from build123d import *

# Parameters (mm, degrees)
SKETCH1_R           = 161.29
BOSS_EXTRUDE1_DEPTH = 161.29
SKETCH3_W           = 4310.634
SKETCH3_H           = 18064.48
SKETCH3_R           = 161.29
BOSS_EXTRUDE3_DEPTH = 161.29
SCALE2_SCALE        = 0.039370079


with BuildPart() as part:
    # Sketch1 → Boss-Extrude1 (new body)
    with BuildSketch(Plane.XY):
        Polygon((-2155.317, 3225.8), (3592.046917484, 8973.163917484), (5747.419448428, 6817.902448428), (2155.317, 3225.8), (2155.317, -3225.8), (-2155.317, -3225.8), align=None)
        with Locations((4804.833357851, 7304.254711836)):
            Circle(SKETCH1_R, mode=Mode.SUBTRACT)
        with Locations((3892.43933595, 6391.860689935)):
            Circle(SKETCH1_R, mode=Mode.SUBTRACT)
        with Locations((2980.04531405, 5479.466668034)):
            Circle(SKETCH1_R, mode=Mode.SUBTRACT)
        with Locations(Location((2253.753739605, 6205.720818177, 0), (0, 0, 180))):
            Circle(SKETCH1_R, mode=Mode.SUBTRACT)
        with Locations(Location((3166.100745307, 7118.161853854, 0), (0, 0, 180))):
            Circle(SKETCH1_R, mode=Mode.SUBTRACT)
        with Locations(Location((4078.447751009, 8030.602889531, 0), (0, 0, 180))):
            Circle(SKETCH1_R, mode=Mode.SUBTRACT)
    extrude(amount=-BOSS_EXTRUDE1_DEPTH)

    # Sketch3 → Boss-Extrude3 (add)
    with BuildSketch(Plane(origin=(0, -3225.8, 0), x_dir=(-1, 0, 0), z_dir=(0, -1, 0))):
        with Locations((0, 9032.24)):
            Rectangle(SKETCH3_W, SKETCH3_H)
        with BuildLine():
            ThreePointArc((-1076.325000002, 3548.374999923), (-961.455647452, 3501.587385122), (-913.765000004, 3387.09))
            ThreePointArc((-913.765000004, 3387.09), (-961.455647452, 3272.592614878), (-1076.325000002, 3225.805000077))
            ThreePointArc((-1076.325000002, 3225.805000077), (-1238.885, 3387.09), (-1076.325000002, 3548.374999923))
        make_face(mode=Mode.SUBTRACT)
        with Locations(Location((1075.054999996, 3387.089999999, 0), (0, 0, 180))):
            Circle(SKETCH3_R, mode=Mode.SUBTRACT)
        with BuildLine():
            ThreePointArc((-1076.325000001, 10322.565000077), (-1238.885, 10483.85), (-1076.325, 10645.134999923))
            ThreePointArc((-1076.325, 10645.134999923), (-961.455647452, 10598.347385122), (-913.765000004, 10483.85))
            ThreePointArc((-913.765000004, 10483.85), (-961.455647452, 10369.352614878), (-1076.325000001, 10322.565000077))
        make_face(mode=Mode.SUBTRACT)
        with BuildLine():
            ThreePointArc((-1076.325000002, 17419.325000077), (-1238.885, 17580.61), (-1076.325000002, 17741.894999923))
            ThreePointArc((-1076.325000002, 17741.894999923), (-961.455647452, 17695.107385122), (-913.765000004, 17580.61))
            ThreePointArc((-913.765000004, 17580.61), (-961.455647452, 17466.112614878), (-1076.325000002, 17419.325000077))
        make_face(mode=Mode.SUBTRACT)
        with Locations(Location((1077.594999996, 10483.849999999, 0), (0, 0, 180))):
            Circle(SKETCH3_R, mode=Mode.SUBTRACT)
        with Locations(Location((1077.595, 17580.609999999, 0), (0, 0, 180))):
            Circle(SKETCH3_R, mode=Mode.SUBTRACT)
    extrude(amount=BOSS_EXTRUDE3_DEPTH)


with BuildPart() as part_1:
    # Scale2: scaled about (342.584657251, -1172.717670217, -5623.777851714)
    add(part.part.scale(SCALE2_SCALE).moved(Location((329.09707232, -1126.547683201, -5402.369274875))))


solid = part_1.part
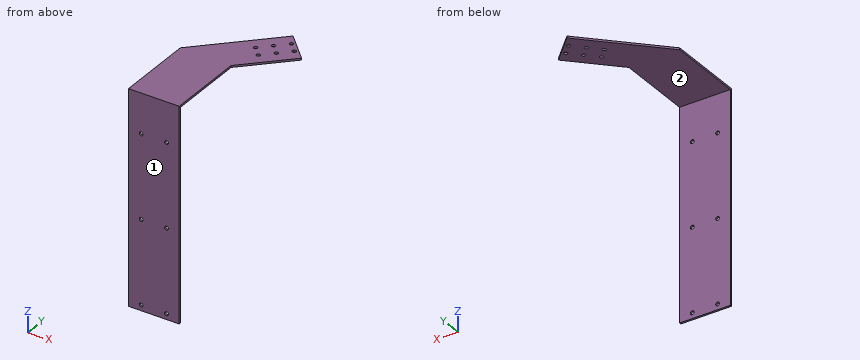
Read the model definition and answer for the solid it produces. Units are mm, in the model's axes. Face numbers are marked on the shaded views. A direction names the side the tool comes from. Round coordinates to 2 decimals unless told otherwise and drop trailing zeros. Write each loop counter-clockwise with the first axis right and the second up, starting at its lowest first coordinate (ties: lowest second). Pieces come first, ordered by that corner, then holes. Notation, with made-up numbers: (-9.75, 69.5) - (13.25, 69.5) arc R14 cw to (13.25, 78.5) - close; hole circle Ø8 at (14, 41). An arc over 180 degrees is marked (long way). Use a Markdown table: item, result.
(1) The part is cut by section A-A (y = -1188). Write down the section's boundary in (x, z).
Reported:
| item | result |
|---|---|
| outline | (244.24, -5408.72) - (413.95, -5408.72) - (413.95, -5402.37) - (244.24, -5402.37) - close |
(2) The part is cut by section D-D (x = 324). Write down the section's boundary in (y, z).
Reported:
| item | result |
|---|---|
| outline | (-1259.9, -6113.57) - (-1253.55, -6113.57) - (-1253.55, -5408.72) - (-919.79, -5408.72) - (-919.79, -5402.37) - (-1259.9, -5402.37) - close |
(3) The part is cut by section C-C (x = 391). Write down the section's boundary in (y, z), then the cut area to 3 significant figures.
Reported:
| item | result |
|---|---|
| outline | (-1259.9, -6113.57) - (-1253.55, -6113.57) - (-1253.55, -5408.72) - (-852.79, -5408.72) - (-852.79, -5402.37) - (-1259.9, -5402.37) - close |
| area | 7,060 mm2 |
(4) Which of the six approach directions +Z, -Z, +X, -X, +Y, -Y give full straight-line access (tool end or side, diameter ignored) to the marked faces 1 and 2?
Reported:
| item | result |
|---|---|
| face 1 | +Z, -Z, +X, -X, -Y |
| face 2 | -Z, +X, -X, +Y |
(5) Straight lines are drawn through the part: line 1 along Y through (x, z) = (309.5, -5901.5); line 2 along Z through (x, y) = (368, -1201). For each, find the intervals that lie inside material, in ascending order. Write a range as [from, to].
Reported:
| item | result |
|---|---|
| line 1 | [-1259.9, -1253.55] |
| line 2 | [-5408.72, -5402.37] |
(6) The part is cut by section B-B (z = -5725). Write down the section's boundary in (x, y).
Reported:
| item | result |
|---|---|
| outline | (244.24, -1259.9) - (413.95, -1259.9) - (413.95, -1253.55) - (244.24, -1253.55) - close |
(7) Each of these flat-tipped pins is pushed along its axis until it touches: pin 1 Ø16.5 at (x, y) = (446.42, -910.82) entering from -Z; pin 2 Ø14.5 at (x, z) = (286.77, -5535.72) entering from +Y. Where does it stop, or does it pass through?
Reported:
| item | result |
|---|---|
| pin 1 | z = -5408.72 |
| pin 2 | y = -1253.55 |
